Read the model definition and answer for the solid it produces. Units are mm, in the model's axes. Face numbers are marked on the shaded views. A direction names the side the tool comes from. Coordinates: 2 decimals unless noted, no trailing zeros. Loops run counter-clockwise (first coordinate to the right, second up) from the corner with the lowest first, then second, coordinate; pieces in that order, holes last. Notation, with made-up numbers: M 72.25,-26.75 L 118.25,-26.75 A19 cw 118.25,-17.75 Z; hole C -13.75,85 d4. An arc over 180 degrees is marked long. Put each result on its own line as item: value.
from build123d import *

# Parameters (mm, degrees)
CROQUIS1_W              = 45
CROQUIS1_H              = 40
SALIENTE_EXTRUIR1_DEPTH = 5
CROQUIS2_W              = 5
CROQUIS2_H              = 40
SALIENTE_EXTRUIR2_DEPTH = 40
CROQUIS13_W             = 40
CROQUIS13_H             = 5
SALIENTE_EXTRUIR7_DEPTH = 40
CORTAR_EXTRUIR3_REACH   = 88.783
CROQUIS15_R             = 12.5
CORTAR_EXTRUIR4_REACH   = 88.783
CROQUIS18_R             = 1.5
CROQUIS24_W             = 5.6
CROQUIS24_H             = 5.7
CROQUIS24_W_2           = 5.7
CROQUIS24_H_2           = 5.6
SALIENTE_EXTRUIR8_DEPTH = 40
CROQUIS20_W             = 40
CROQUIS20_H             = 6.2
CORTAR_EXTRUIR5_DEPTH   = 5.7
CROQUIS21_W             = 40
CROQUIS21_H             = 6.2
CORTAR_EXTRUIR6_DEPTH   = 5.7
CORTAR_EXTRUIR7_REACH   = 68.708
CROQUIS22_R             = 2.5
CORTAR_EXTRUIR8_REACH   = 78.852
CROQUIS23_R             = 2.5
REDONDEO1_R             = 10
REDONDEO2_R             = 10


with BuildPart() as part:
    # Croquis1 → Saliente-Extruir1 (new body)
    with BuildSketch(Plane.XY):
        Rectangle(CROQUIS1_W, CROQUIS1_H)
    extrude(amount=SALIENTE_EXTRUIR1_DEPTH)

    # Croquis2 → Saliente-Extruir2 (add)
    with BuildSketch(Plane.XY.offset(5)):
        with Locations((20, 0)):
            Rectangle(CROQUIS2_W, CROQUIS2_H)
    extrude(amount=SALIENTE_EXTRUIR2_DEPTH)

    # Croquis13 → Saliente-Extruir7 (add)
    with BuildSketch(Plane(origin=(22.5, 0, 0), x_dir=(0, 0, -1), z_dir=(1, 0, 0))):
        with Locations((15, 17.5)):
            Rectangle(CROQUIS13_W, CROQUIS13_H)
    extrude(amount=SALIENTE_EXTRUIR7_DEPTH)

    # Croquis15 → Cortar-Extruir3 (cut, up to next)
    with BuildSketch(Plane(origin=(0, 20, 0), x_dir=(1, 0, 0), z_dir=(0, 1, 0)), mode=Mode.PRIVATE) as cortar_extruir3_sk1:
        with Locations(Location((42.5, 15, 0), (0, 0, 180))):
            Circle(CROQUIS15_R)
    cortar_extruir3_tool1 = extrude(cortar_extruir3_sk1.sketch, amount=-CORTAR_EXTRUIR3_REACH, mode=Mode.PRIVATE) & part.part
    add(cortar_extruir3_tool1.solids().sort_by_distance((42.5, 20, -15))[0], mode=Mode.SUBTRACT)

    # Croquis18 → Cortar-Extruir4 (cut, up to next)
    with BuildSketch(Plane(origin=(0, 20, 0), x_dir=(1, 0, 0), z_dir=(0, 1, 0)), mode=Mode.PRIVATE) as cortar_extruir4_sk1:
        with Locations(Location((27, 30.5, 0), (0, 0, 180))):
            Circle(CROQUIS18_R)
    cortar_extruir4_tool1 = extrude(cortar_extruir4_sk1.sketch, amount=-CORTAR_EXTRUIR4_REACH, mode=Mode.PRIVATE) & part.part
    # Croquis18 → Cortar-Extruir4 (cut, up to next)
    with BuildSketch(Plane(origin=(0, 20, 0), x_dir=(1, 0, 0), z_dir=(0, 1, 0)), mode=Mode.PRIVATE) as cortar_extruir4_sk2:
        with Locations(Location((58, 30.5, 0), (0, 0, 180))):
            Circle(CROQUIS18_R)
    cortar_extruir4_tool2 = extrude(cortar_extruir4_sk2.sketch, amount=-CORTAR_EXTRUIR4_REACH, mode=Mode.PRIVATE) & part.part
    # Croquis18 → Cortar-Extruir4 (cut, up to next)
    with BuildSketch(Plane(origin=(0, 20, 0), x_dir=(1, 0, 0), z_dir=(0, 1, 0)), mode=Mode.PRIVATE) as cortar_extruir4_sk3:
        with Locations(Location((58, -0.5, 0), (0, 0, 180))):
            Circle(CROQUIS18_R)
    cortar_extruir4_tool3 = extrude(cortar_extruir4_sk3.sketch, amount=-CORTAR_EXTRUIR4_REACH, mode=Mode.PRIVATE) & part.part
    # Croquis18 → Cortar-Extruir4 (cut, up to next)
    with BuildSketch(Plane(origin=(0, 20, 0), x_dir=(1, 0, 0), z_dir=(0, 1, 0)), mode=Mode.PRIVATE) as cortar_extruir4_sk4:
        with Locations(Location((27, -0.5, 0), (0, 0, 180))):
            Circle(CROQUIS18_R)
    cortar_extruir4_tool4 = extrude(cortar_extruir4_sk4.sketch, amount=-CORTAR_EXTRUIR4_REACH, mode=Mode.PRIVATE) & part.part
    add(cortar_extruir4_tool1.solids().sort_by_distance((27, 20, -30.5))[0], mode=Mode.SUBTRACT)
    add(cortar_extruir4_tool2.solids().sort_by_distance((58, 20, -30.5))[0], mode=Mode.SUBTRACT)
    add(cortar_extruir4_tool3.solids().sort_by_distance((58, 20, 0.5))[0], mode=Mode.SUBTRACT)
    add(cortar_extruir4_tool4.solids().sort_by_distance((27, 20, 0.5))[0], mode=Mode.SUBTRACT)

    # Croquis24 → Saliente-Extruir8 (add)
    with BuildSketch(Plane(origin=(0, -20, 0), x_dir=(-1, 0, 0), z_dir=(0, -1, 0))):
        with Locations((12.5, -7.85)):
            Rectangle(CROQUIS24_W, CROQUIS24_H)
        with Locations((-7.5, -7.85)):
            Rectangle(CROQUIS24_W, CROQUIS24_H)
        with Locations((-14.65, -35)):
            Rectangle(CROQUIS24_W_2, CROQUIS24_H_2)
        with Locations((-14.65, -15)):
            Rectangle(CROQUIS24_W_2, CROQUIS24_H_2)
    extrude(amount=-SALIENTE_EXTRUIR8_DEPTH)

    # Croquis20 → Cortar-Extruir5 (cut)
    with BuildSketch(Plane.ZY.offset(-11.8)):
        with Locations((25, -12.6)):
            Rectangle(CROQUIS20_W, CROQUIS20_H)
        with Locations((25, 12.6)):
            Rectangle(CROQUIS20_W, CROQUIS20_H)
    extrude(amount=-CORTAR_EXTRUIR5_DEPTH, mode=Mode.SUBTRACT)

    # Croquis21 → Cortar-Extruir6 (cut)
    with BuildSketch(Plane.XY.offset(10.7)):
        with Locations((-2.5, -12.6)):
            Rectangle(CROQUIS21_W, CROQUIS21_H)
        with Locations((-2.5, 11.7)):
            Rectangle(CROQUIS21_W, CROQUIS21_H)
    extrude(amount=-CORTAR_EXTRUIR6_DEPTH, mode=Mode.SUBTRACT)

    # Croquis22 → Cortar-Extruir7 (cut, up to next)
    with BuildSketch(Plane.ZY.offset(-17.5), mode=Mode.PRIVATE) as cortar_extruir7_sk1:
        with Locations(Location((15, 13.05, 0), (0, 0, 270))):
            Circle(CROQUIS22_R)
    cortar_extruir7_tool1 = extrude(cortar_extruir7_sk1.sketch, amount=-CORTAR_EXTRUIR7_REACH, mode=Mode.PRIVATE) & part.part
    # Croquis22 → Cortar-Extruir7 (cut, up to next)
    with BuildSketch(Plane.ZY.offset(-17.5), mode=Mode.PRIVATE) as cortar_extruir7_sk2:
        with Locations(Location((35, 13.05, 0), (0, 0, 270))):
            Circle(CROQUIS22_R)
    cortar_extruir7_tool2 = extrude(cortar_extruir7_sk2.sketch, amount=-CORTAR_EXTRUIR7_REACH, mode=Mode.PRIVATE) & part.part
    # Croquis22 → Cortar-Extruir7 (cut, up to next)
    with BuildSketch(Plane.ZY.offset(-17.5), mode=Mode.PRIVATE) as cortar_extruir7_sk3:
        with Locations(Location((15, -13.05, 0), (0, 0, 270))):
            Circle(CROQUIS22_R)
    cortar_extruir7_tool3 = extrude(cortar_extruir7_sk3.sketch, amount=-CORTAR_EXTRUIR7_REACH, mode=Mode.PRIVATE) & part.part
    # Croquis22 → Cortar-Extruir7 (cut, up to next)
    with BuildSketch(Plane.ZY.offset(-17.5), mode=Mode.PRIVATE) as cortar_extruir7_sk4:
        with Locations(Location((35, -13.05, 0), (0, 0, 270))):
            Circle(CROQUIS22_R)
    cortar_extruir7_tool4 = extrude(cortar_extruir7_sk4.sketch, amount=-CORTAR_EXTRUIR7_REACH, mode=Mode.PRIVATE) & part.part
    add(cortar_extruir7_tool1.solids().sort_by_distance((17.5, 13.05, 15))[0], mode=Mode.SUBTRACT)
    add(cortar_extruir7_tool2.solids().sort_by_distance((17.5, 13.05, 35))[0], mode=Mode.SUBTRACT)
    add(cortar_extruir7_tool3.solids().sort_by_distance((17.5, -13.05, 15))[0], mode=Mode.SUBTRACT)
    add(cortar_extruir7_tool4.solids().sort_by_distance((17.5, -13.05, 35))[0], mode=Mode.SUBTRACT)

    # Croquis23 → Cortar-Extruir8 (cut, up to next)
    with BuildSketch(Plane.XY.offset(5), mode=Mode.PRIVATE) as cortar_extruir8_sk1:
        with Locations((-12.5, 12.15)):
            Circle(CROQUIS23_R)
    cortar_extruir8_tool1 = extrude(cortar_extruir8_sk1.sketch, amount=-CORTAR_EXTRUIR8_REACH, mode=Mode.PRIVATE) & part.part
    # Croquis23 → Cortar-Extruir8 (cut, up to next)
    with BuildSketch(Plane.XY.offset(5), mode=Mode.PRIVATE) as cortar_extruir8_sk2:
        with Locations((7.5, 12.15)):
            Circle(CROQUIS23_R)
    cortar_extruir8_tool2 = extrude(cortar_extruir8_sk2.sketch, amount=-CORTAR_EXTRUIR8_REACH, mode=Mode.PRIVATE) & part.part
    # Croquis23 → Cortar-Extruir8 (cut, up to next)
    with BuildSketch(Plane.XY.offset(5), mode=Mode.PRIVATE) as cortar_extruir8_sk3:
        with Locations((-12.5, -13.05)):
            Circle(CROQUIS23_R)
    cortar_extruir8_tool3 = extrude(cortar_extruir8_sk3.sketch, amount=-CORTAR_EXTRUIR8_REACH, mode=Mode.PRIVATE) & part.part
    # Croquis23 → Cortar-Extruir8 (cut, up to next)
    with BuildSketch(Plane.XY.offset(5), mode=Mode.PRIVATE) as cortar_extruir8_sk4:
        with Locations((7.5, -13.05)):
            Circle(CROQUIS23_R)
    cortar_extruir8_tool4 = extrude(cortar_extruir8_sk4.sketch, amount=-CORTAR_EXTRUIR8_REACH, mode=Mode.PRIVATE) & part.part
    add(cortar_extruir8_tool1.solids().sort_by_distance((-12.5, 12.15, 5))[0], mode=Mode.SUBTRACT)
    add(cortar_extruir8_tool2.solids().sort_by_distance((7.5, 12.15, 5))[0], mode=Mode.SUBTRACT)
    add(cortar_extruir8_tool3.solids().sort_by_distance((-12.5, -13.05, 5))[0], mode=Mode.SUBTRACT)
    add(cortar_extruir8_tool4.solids().sort_by_distance((7.5, -13.05, 5))[0], mode=Mode.SUBTRACT)

    # Redondeo1
    # the kernel refuses this fillet: 10 mm, written as the material it adds along each edge
    with BuildSketch(Plane(origin=(22.5, 20, 5), x_dir=(0, 0, 1), z_dir=(0, -1, 0))) as redondeo1_piece_1_section:
        with BuildLine():
            CenterArc((REDONDEO1_R, -REDONDEO1_R), REDONDEO1_R, 90, 90)
            Line((0, -REDONDEO1_R), (0, 0))
            Line((0, 0), (REDONDEO1_R, 0))
        make_face()
    redondeo1_piece_1 = extrude(amount=5, mode=Mode.PRIVATE)
    redondeo1_piece_1 = redondeo1_piece_1 - Plane(origin=(24.766392733, 13.05, 15), x_dir=(0, -1, 0), z_dir=(-1, 0, 0)) * Cylinder(2.5, 50, mode=Mode.PRIVATE)
    add(redondeo1_piece_1)

    # Redondeo2
    redondeo2_edges = [part.edges().sort_by_distance(p)[0] for p in [
        (22.5, 17.5, 0),
    ]]
    fillet(redondeo2_edges, radius=REDONDEO2_R)


solid = part.part
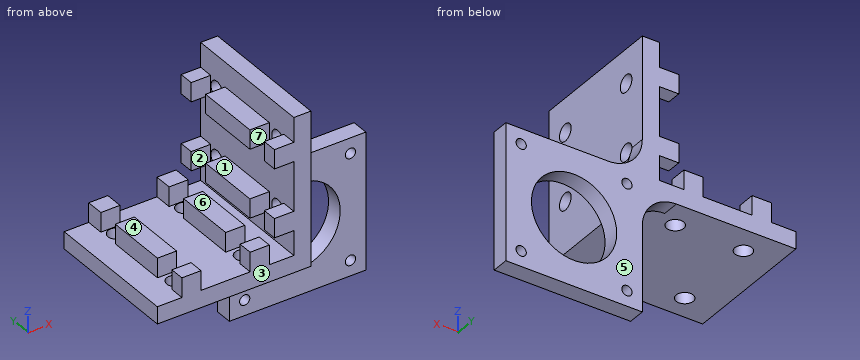
1) Find section A-A, the plane x = -12.5. Write down the section's boundary in (y, z), plus the area to 3 significant figures.
Answer list:
outline: M -20,0 L -15.55,0 L -15.55,5 L -15.7,5 L -15.7,10.7 L -20,10.7 Z; M -10.55,0 L 9.65,0 L 9.65,5 L 8.6,5 L 8.6,10.7 L -9.5,10.7 L -9.5,5 L -10.55,5 Z; M 14.65,0 L 20,0 L 20,10.7 L 14.8,10.7 L 14.8,5 L 14.65,5 Z
area: 307 mm^2
2) Determine the mould class of the marked faces 5, 6 and 7 for opening direction Y: released by +Y, released by -Y, zero draft, split by the parting line, or undercut.
Answer list:
face 5: released by +Y
face 6: zero draft
face 7: undercut
3) Given pin 1 Ø2.5 at (x, z) = (27, 0.5) entering from +Y; pin 2 Ø8 at (y, z) = (2.5, 0.5) entering from +X; pin 3 Ø2.5 at (y, z) = (18.5, 6.5) entering from -X; pin 4 Ø4.5 at (x, y) = (14, 17.5) entering from -Z, each flat-ended and moving along its own axis, determine where each tip first touches the part or whether it passes through.
Answer list:
pin 1: passes through
pin 2: stops at x = 22.5
pin 3: stops at x = -15.3
pin 4: stops at z = -0.73
4) Which of the six approach directions +Z, -Z, +X, -X, +Y, -Y give full straight-line access (tool end or side, diameter ignored) to the marked faces 1, 2, 3 and 4?
Answer list:
face 1: -X, +Y, -Y
face 2: +Z, -X
face 3: +Z, -Z, +X, -X, -Y
face 4: +Z, -X, +Y, -Y
5) Find section B-B, the plane z = -15. Write down the section's boundary in (x, y).
Answer list:
outline: M 22.5,15 L 30,15 L 30,20 L 22.5,20 Z; M 55,15 L 62.5,15 L 62.5,20 L 55,20 Z
6) Find section C-C, the plane y = -13.05. Write down the section's boundary in (x, z).
Answer list:
outline: M -22.5,0 L -15,0 L -15,5 L -22.5,5 Z; M -10,0 L 5,0 L 5,5 L -10,5 Z; M 10,0 L 22.5,0 L 22.5,12.5 L 17.5,12.5 L 17.5,5 L 10,5 Z; M 17.5,17.5 L 22.5,17.5 L 22.5,32.5 L 17.5,32.5 Z; M 17.5,37.5 L 22.5,37.5 L 22.5,45 L 17.5,45 Z
7) Straight lines are drawn through the part: line 1 (Z direction, x = 19.2, y = 13.05); line 2 (Y direction, x = -12.5, z = 2.65); line 3 (Z direction, x = 58, y = 17.1). For each, find the intervals that lie inside material, in ascending order. Write a range as [from, to].
Answer list:
line 1: z = [0, 12.5], [17.5, 32.5], [37.5, 45]
line 2: y = [-20, -15.55], [-10.55, 9.65], [14.65, 20]
line 3: z = [-35, -32], [-29, -1], [2, 5]
8) Find section D-D, the plane x = 42.5. Write down the section's boundary in (y, z), plus the area to 3 significant figures.
Answer list:
outline: M 15,-35 L 20,-35 L 20,-27.5 L 15,-27.5 Z; M 15,-2.5 L 20,-2.5 L 20,5 L 15,5 Z
area: 75.0 mm^2
